Geometry: final body of the model. Coordinates: model frame, mm. A direction names the side the tool comes from. Coordinates: 2 decimals unless noted, no trailing zeros. Loops run counter-clockwise (first coordinate to the right, second up) from the corner with the lowest first, then second, coordinate; pieces in that order, holes last. Notation, with made-up numbers: (-14.5, 42) - (-7.5, 42) arc R24 ccw to (-7.5, 75) - close; hole circle Ø10 at (32.25, 53.25). An arc over 180 degrees is marked (long way). Put each result on its own line as item: value. Start each with the question number.
1) Section C-C on x = 346. Output: boundary loops of the cut face in (y, z), and give its area (3 significant figures).
2) Draft query along Y for faces 1 (the flat face through (12, -474, 0.452)), 2 (the flat face through (283, -286, 352.552)), 3 (the flat face through (12, 393.7, 174)). Return one class per face: +Y half, -Y half, draft (parallel to the pull), parting line (faces both ways), or undercut.
3) Reachability of faces 4 (the flat face through (283, 286, 352.552)), 5 (the flat face through (-84, 381, 179)), 6 (the flat face through (12, 474, 12.7)), 7 (the flat face through (-873.125, 195, 347)) from +Z, -Z, +X, -X, +Y, -Y: full face, straight path, thin tool, end or side. Return the list, or none.
4) Material intervals for line 1 along X through (y, z) = (285, 367) (3 decimals); line 2 along Y through (x, z) = (-157.5, 42); line 3 along Z through (x, y) = (-425, 471), sorted ascending. Write a range as from..to.
5) Section B-B on z = 61.5. Output: boundary loops of the cut face in (x, y) (3 decimals), and give its area (3 significant figures).
6) Contact query for flat-ended pins moving along their axis: pin 1 Ø3 at (x, y) = (-449.5, 385) entering from +Z; pin 2 Ø10 at (y, z) = (130.5, 119) entering from -X (3 decimals); pin 3 Ø12 at (y, z) = (-112.5, 322.5) entering from +X (3 decimals). Output: stop coordinate, or through.
7) Section A-A on y = -285.75. Output: boundary loops of the cut face in (x, z) (1 decimal).
8) Section D-D on y = 93.5. Output: boundary loops of the cut face in (x, z) (3 decimals).
```python
from build123d import *

# Parameters (mm, degrees)
F1_DEPTH = 873.125
F2_W     = 12.7
F2_H     = 762
F3_DEPTH = 339.400452
F4_W     = 234.95
F4_H     = 171.45
F4_R     = 17.4625
F4_W_2   = 304.8
F5_DEPTH = 25.4


with BuildPart() as f1:
    # F0 (on Right) → F1 (new body, symmetric)
    with BuildSketch(Plane.YZ):
        with BuildLine():
            Line((0, 339.852), (0, 352.552))
            Line((0, 352.552), (-361.95, 352.552))
            ThreePointArc((-361.95, 352.552), (-384.40064, 343.25264), (-393.7, 320.802))
            Line((-393.7, 320.802), (-393.7, 31.75))
            ThreePointArc((-393.7, 31.75), (-399.279616, 18.279616), (-412.75, 12.7))
            Line((-412.75, 12.7), (-516.630888, 12.7))
            Line((-516.630888, 12.7), (-520.7, 12.7))
            Line((-520.7, 12.7), (-533.4, 12.7))
            Line((-533.4, 12.7), (-533.4, 0.451548))
            Line((-533.4, 0.451548), (-412.75, 0.451548))
            ThreePointArc((-412.75, 0.451548), (-390.29936, 9.750908), (-381, 32.201548))
            Line((-381, 32.201548), (-381, 320.802))
            ThreePointArc((-381, 320.802), (-375.420384, 334.272384), (-361.95, 339.852))
            Line((-361.95, 339.852), (0, 339.852))
        make_face()
        with BuildLine():
            Line((361.95, 352.552), (0, 352.552))
            Line((0, 352.552), (0, 339.852))
            Line((0, 339.852), (361.95, 339.852))
            ThreePointArc((361.95, 339.852), (375.420384, 334.272384), (381, 320.802))
            Line((381, 320.802), (381, 32.201548))
            ThreePointArc((381, 32.201548), (390.29936, 9.750908), (412.75, 0.451548))
            Line((412.75, 0.451548), (533.4, 0.451548))
            Line((533.4, 0.451548), (533.4, 12.7))
            Line((533.4, 12.7), (520.7, 12.7))
            Line((520.7, 12.7), (516.630888, 12.7))
            Line((516.630888, 12.7), (412.75, 12.7))
            ThreePointArc((412.75, 12.7), (399.279616, 18.279616), (393.7, 31.75))
            Line((393.7, 31.75), (393.7, 320.802))
            ThreePointArc((393.7, 320.802), (384.40064, 343.25264), (361.95, 352.552))
        make_face()
    extrude(amount=F1_DEPTH, both=True)

    # F2 (on face) → F3 (join, through all)
    with BuildSketch(Plane(origin=(0, 0, 339.852), x_dir=(1, 0, 0), z_dir=(0, 0, -1))):
        with Locations((688.975, 0)):
            Rectangle(F2_W, F2_H)
    extrude(amount=F3_DEPTH)

    # F4 (on face) → F5 (join)
    with BuildSketch(Plane.XY.offset(352.552)):
        with Locations((-431.8, 269.875)):
            Rectangle(F4_W, F4_H)
        with Locations((-441.325, 285.75)):
            Circle(F4_R, mode=Mode.SUBTRACT)
        with Locations((238.125, 269.875)):
            Rectangle(F4_W_2, F4_H)
        with Locations((282.575, 285.75)):
            Circle(F4_R, mode=Mode.SUBTRACT)
        with Locations((238.125, -269.875)):
            Rectangle(F4_W_2, F4_H)
        with Locations((282.575, -285.75)):
            Circle(F4_R, mode=Mode.SUBTRACT)
        with Locations((-431.8, -269.875)):
            Rectangle(F4_W, F4_H)
        with Locations((-441.325, -285.75)):
            Circle(F4_R, mode=Mode.SUBTRACT)
    extrude(amount=F5_DEPTH)


solid = f1.part
```
Answer block:
1. outline: (-533.4, 0.45) - (-412.75, 0.45) arc R31.75 ccw to (-381, 32.2) - (-381, 320.8) arc R19.05 cw to (-361.95, 339.85) - (361.95, 339.85) arc R19.05 cw to (381, 320.8) - (381, 32.2) arc R31.75 ccw to (412.75, 0.45) - (533.4, 0.45) - (533.4, 12.7) - (412.75, 12.7) arc R19.05 cw to (393.7, 31.75) - (393.7, 320.8) arc R31.75 ccw to (361.95, 352.55) - (355.6, 352.55) - (355.6, 377.95) - (184.15, 377.95) - (184.15, 352.55) - (-184.15, 352.55) - (-184.15, 377.95) - (-355.6, 377.95) - (-355.6, 352.55) - (-361.95, 352.55) arc R31.75 ccw to (-393.7, 320.8) - (-393.7, 31.75) arc R19.05 cw to (-412.75, 12.7) - (-533.4, 12.7) - close
1. area: 30,200 mm²
2. face 1: draft
2. face 2: undercut
2. face 3: +Y half
3. face 4: +Z
3. face 5: -Z, -X
3. face 6: +Z, +X, -X, +Y
3. face 7: +Z, -Z, -X, +Y, -Y
4. line 1: x = -549.275..-458.771, -423.879..-314.325, 85.725..265.129, 300.021..390.525
4. line 2: y = -393.7..-381, 381..393.7
4. line 3: z = 0.45..12.7
5. outline: (-873.125, -393.7) - (873.125, -393.7) - (873.125, -381) - (695.325, -381) - (695.325, 381) - (873.125, 381) - (873.125, 393.7) - (-873.125, 393.7) - (-873.125, 381) - (682.625, 381) - (682.625, -381) - (-873.125, -381) - close
5. area: 54,000 mm²
6. pin 1: stops at z = 344.12
6. pin 2: stops at x = 682.625
6. pin 3: stops at x = 695.325
7. outline: (-873.1, 339.9) - (682.6, 339.9) - (682.6, 0.5) - (695.3, 0.5) - (695.3, 339.9) - (873.1, 339.9) - (873.1, 352.6) - (390.5, 352.6) - (390.5, 378) - (300, 378) - (300, 352.6) - (265.1, 352.6) - (265.1, 378) - (85.7, 378) - (85.7, 352.6) - (-314.3, 352.6) - (-314.3, 378) - (-423.9, 378) - (-423.9, 352.6) - (-458.8, 352.6) - (-458.8, 378) - (-549.3, 378) - (-549.3, 352.6) - (-873.1, 352.6) - close
8. outline: (-873.125, 339.852) - (682.625, 339.852) - (682.625, 0.452) - (695.325, 0.452) - (695.325, 339.852) - (873.125, 339.852) - (873.125, 352.552) - (-873.125, 352.552) - close
